```python
from build123d import *

# Parameters (mm, degrees)
SKETCH1_R           = 43.18
BOSS_EXTRUDE1_DEPTH = 9.271


with BuildPart() as part:
    # Sketch1 → Boss-Extrude1 (new body)
    with BuildSketch(Plane.XY):
        Circle(SKETCH1_R)
        with BuildLine():
            Line((4.501497694, 5.157177285), (6.716995387, 1.319822715))
            ThreePointArc((6.716995387, 1.319822715), (8.240995387, 1.319822715), (9.002995387, 0))
            ThreePointArc((9.002995387, 0), (8.240995387, -1.319822715), (6.716995387, -1.319822715))
            Line((6.716995387, -1.319822715), (4.501497694, -5.157177285))
            ThreePointArc((4.501497694, -5.157177285), (5.059320409, -5.715), (5.263497694, -6.477))
            ThreePointArc((5.263497694, -6.477), (3.739497694, -8.001), (2.215497694, -6.477))
            Line((2.215497694, -6.477), (-2.215497694, -6.477))
            ThreePointArc((-2.215497694, -6.477), (-4.501497694, -7.796822715), (-4.501497694, -5.157177285))
            Line((-4.501497694, -5.157177285), (-6.716995387, -1.319822715))
            ThreePointArc((-6.716995387, -1.319822715), (-9.002995387, 0), (-6.716995387, 1.319822715))
            Line((-6.716995387, 1.319822715), (-4.501497694, 5.157177285))
            ThreePointArc((-4.501497694, 5.157177285), (-4.501497694, 7.796822715), (-2.215497694, 6.477))
            Line((-2.215497694, 6.477), (2.215497694, 6.477))
            ThreePointArc((2.215497694, 6.477), (3.739497694, 8.001), (5.263497694, 6.477))
            ThreePointArc((5.263497694, 6.477), (5.059320409, 5.715), (4.501497694, 5.157177285))
        make_face(mode=Mode.SUBTRACT)
    extrude(amount=BOSS_EXTRUDE1_DEPTH)


solid = part.part
```
Work out the finished part from the listing and answer in its coordinate system (mm). A direction names the side the tool comes from. Give positions to 0.01 mm unless a question says otherwise; leave off trailing zeros. Loops run counter-clockwise (first coordinate to the right, second up) from the corner with the lowest first, then second, coordinate; pieces in that order, holes last. Notation, with made-up numbers: (86.25, 34) -> (102.25, 34) arc R17 cw to (102.25, 53) -> close; hole circle Ø10 at (-35, -20.5). An arc over 180 degrees is marked (long way). One line per question, with ' | ' between items. Start each with the question number.
1) Section B-B, the plane z = 1.25 is taken. Determine the outline of the cut face in (x, y), then the cut area to 3 significant figures.
2) Section D-D, the plane x = 23.5 is taken. Determine the outline of the cut face in (y, z).
3) Straight lines are drawn through the part: L1, parallel to Y at x = 0, z = 5.25; L2, parallel to Y at x = 6, z = 2.75; L3, parallel to X at y = 5, z = 7. For each, find the intervals that lie inside material, in ascending order.
4) For faces 5 (the face through (-1, -9, 9.271)), 6 (the face through (-5.625, 3.212, 4.571)), determine the directions among +Z, -Z, +X, -X, +Y, -Y from which every point of the face is accessible in a straight line to the end or side of a thin tool.
5) Section A-A, the plane x = 0 is taken. Determine the outline of the cut face in (y, z), then the cut area to 3 significant figures.
6) Each of these flat-tipped pins is pushed along its axis until it touches: pin 1 (3.5 mm diameter, centred on x = -3.74, y = 6.48, fed in from -Z); pin 2 (3 mm diameter, centred on y = 16, z = 6.5, fed in from -X); pin 3 (5 mm diameter, centred on x = -24.5, z = 4.5, fed in from -Y); pin 4 (1 mm diameter, centred on x = -15.5, z = 3.5, fed in from -Y). Where does it stop, or does it pass through?
7) Section C-C, the plane y = 28.5 is taken. Determine the outline of the cut face in (x, z), then the cut area to 3 significant figures.
8) Determine the mould class of faces 1 (the face through (5.625, -3.212, 4.571)), 2 (the face through (-4.54, 7.774, 4.571)), 3 (the face through (-31.83, 29.18, 4.57)), 4 (the face through (-1, -9, 0)) for opening direction X: +X half, -X half, draft (parallel to the pull), parting line (faces both ways), or undercut.
Resolved:
1) outline: circle Ø86.36 at (0, 0); hole (-6.72, -1.32) -> (-4.5, -5.16) arc R1.52 ccw (long way) to (-2.22, -6.48) -> (2.22, -6.48) arc R1.52 ccw (long way) to (4.5, -5.16) -> (6.72, -1.32) arc R1.52 ccw (long way) to (6.72, 1.32) -> (4.5, 5.16) arc R1.52 ccw (long way) to (2.22, 6.48) -> (-2.22, 6.48) arc R1.52 ccw (long way) to (-4.5, 5.16) -> (-6.72, 1.32) arc R1.52 ccw (long way) to start | area: 5,680 mm2
2) outline: (-36.23, 0) -> (36.23, 0) -> (36.23, 9.27) -> (-36.23, 9.27) -> close
3) L1: -43.18 to -6.48, 6.48 to 43.18 | L2: -42.76 to -2.56, 2.56 to 42.76 | L3: -42.89 to -4.59, 4.59 to 42.89
4) face 5: +Z, +X, -X, +Y, -Y | face 6: +Z, -Z
5) outline: (-43.18, 0) -> (-6.48, 0) -> (-6.48, 9.27) -> (-43.18, 9.27) -> close; (6.48, 0) -> (43.18, 0) -> (43.18, 9.27) -> (6.48, 9.27) -> close | area: 681 mm2
6) pin 1: z = 0 | pin 2: x = -40.67 | pin 3: y = -37.16 | pin 4: y = -40.49
7) outline: (-32.44, 0) -> (32.44, 0) -> (32.44, 9.27) -> (-32.44, 9.27) -> close | area: 601 mm2
8) face 1: undercut | face 2: undercut | face 3: parting line | face 4: draft
